Design review of the part built by this model. Coordinates are the model's own, in mm. Face numbers are marked on the shaded views. A direction names the side the tool comes from. Coordinates: 2 decimals unless noted, no trailing zeros. Order: outer loops, then holes, each group sorted by start corner. A loop starts at its lowest first (then second) coordinate and runs counter-clockwise, first axis right, second up. Notation, with made-up numbers: M 21,83 L 75,83 A10 cw 75,96 Z; hole C 61,-1 d8. An arc over 180 degrees is marked long. Use CSV: the item, a comma, the result in double quotes.
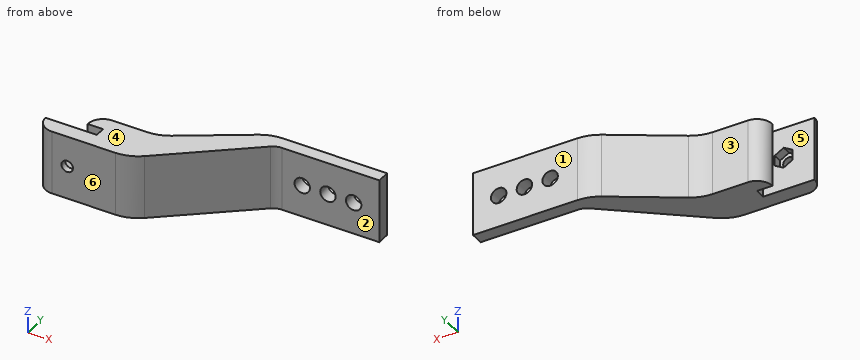
Autodesk Fusion 360 part; units mm, degrees
sketch "Sketch1" plane through (0, 0, 0) normal (0, 0, 1) x (1, 0, 0)
  line L0 (0, 0) -> (0, 6)
  line L1 (0, 6) -> (20, 6)
  line L2 (20, 6) -> (20, 10)
  line L3 (20, 10) -> (14, 10)
  line L4 (14, 16) -> (14, 10)
  line L5 (14, 16) -> (38, 16)
  line L6 (38, 16) -> (70, 36)
  line L7 (70, 36) -> (115, 36)
  line L8 (115, 36) -> (115, 31)
  line L9 (115, 31) -> (75, 31)
  line L10 (75, 31) -> (36, 0)
  line L11 (36, 0) -> (0, 0)
  dimension "d1" = 4
  dimension "d2" = 24
  dimension "d6" = 115
  dimension "d7" = 5
  dimension "d8" = 45
  dimension "d10" = 20
  dimension "d11" = 36
  dimension "d12" = 16
  dimension "d13" = 6
  dimension "d14" = 14
  dimension "d15" = 36
  dimension "d16" = 40
extrude "Extrude1" add sketch "Sketch1" along normal blind 25
sketch "Sketch2" plane through (0, 6, 0) normal (0, 1, 0) x (-1, 0, 0)
  line L0 (-20, 0) -> (0, 0)
  line L1 (0, 0) -> (0, 25)
  line L2 (0, 25) -> (-20, 25)
  line L3 (-20, 25) -> (-20, 0)
  line L4 (0, 13) -> (-20, 13) construction
  line L5 (-12, 25) -> (-12, 0) construction
  line L6 (-8.5, 15.0207) -> (-12, 17.0415)
  line L7 (-12, 17.0415) -> (-15.5, 15.0207)
  line L8 (-15.5, 15.0207) -> (-15.5, 10.9793)
  line L9 (-15.5, 10.9793) -> (-12, 8.9585)
  line L10 (-12, 8.9585) -> (-8.5, 10.9793)
  line L11 (-8.5, 10.9793) -> (-8.5, 15.0207)
  point P0 (-12, 13)
  dimension "d19" = 12
  dimension "d20" = 3.5
extrude "Extrude2" cut sketch "Sketch2" against normal blind 3.5 contours L6 L7 L8 L9 L10 L11
hole "Hole1" at (12, 6, 13) direction (0, -1, 0) diameter 4.5 end through all
sketch "Sketch3" plane through (0, 36, 0) normal (0, 1, 0) x (-1, 0, 0)
  line L0 (-115, 0) -> (-70, 0)
  line L1 (-70, 0) -> (-70, 25)
  line L2 (-70, 25) -> (-115, 25)
  line L3 (-115, 25) -> (-115, 0)
  line L4 (-115, 12.5) -> (-70, 12.5) construction
  line L5 (-105, 25) -> (-105, 0) construction
  point P0 (-105, 12.5)
  dimension "d26" = 10
hole "Hole2" at (105, 36, 12.5) direction (0, -1, 0) diameter 6 depth 6.5 tip angle 118
pattern_linear "R-Pattern1" count 3 spacing 10 along (-1, 0, 0) of "Hole2"
fillet "Fillet1" radius 15 1 edges at (70, 36, 12.5)
fillet "Fillet1" radius 6 1 edges at (75, 31, 12.5)
fillet "Fillet2" radius 15 2 edges at (38, 16, 12.5) (36, 0, 12.5)
fillet "Fillet3" radius 6 1 edges at (14, 16, 12.5)
fillet "Fillet4" radius 6 1 edges at (0, 0, 12.5)
(1) The part is to be moulded in two halves that separate along Y. For the marked faces 4, 5 and 6, say which applies: pulls with the +Y half, pulls with the -Y half, needs draft (parallel to the pull), parting line crosses it, or undercut.
The answers:
face 4,"needs draft"
face 5,"undercut"
face 6,"pulls with the -Y half"
(2) Wall thickness on probe 1 along Z at (x, y) = (95, 33); probe 2 along Z at (x, y) = (12, 1); probe 3 along X at (y, z) = (33.95, 12.5): over which ranges is each line inside the solid? List them lowest first.
The answers:
probe 1,"z = 0 to 9.5, 15.5 to 25"
probe 2,"z = 0 to 10.75, 15.25 to 25"
probe 3,"x = 66.73 to 82, 88 to 92, 98 to 102, 108 to 115"
(3) For the marked faces 1, 2 and 3, list the 3-axis set-ups (+Z, -Z, +X, -X, +Y, -Y) from which the entire face can be reached by the end or side of a thin tool; tool diameter is ignored.
The answers:
face 1,"+Z, -Z, +X, -X, +Y"
face 2,"+Z, -Z, +X, -Y"
face 3,"+Z, -Z, -X, +Y"
(4) Add section D-D on z = 12.5. Give the number of separate pieces and of enclosed holes in the cut face, and give its area (3 significant figures).
The answers:
separate pieces,"5"
enclosed holes,"0"
area,"908 mm2"
(5) Add section B-B on y = 32. State the section outline as (x, z) points, and give its area (3 significant figures).
The answers:
outline,"M 63.6,0 L 115,0 L 115,25 L 63.6,25 Z; hole C 85,12.5 d6; hole C 95,12.5 d6; hole C 105,12.5 d6"
area,"1,200 mm2"
(6) Clearance check with flat-ended pins moving along their axes: P1, Ø8, axis at x = 69.5, z = 6, coming from the +Y side; P2, Ø1, axis at x = 42, z = 3, coming from the +Y side; P3, Ø1.5, axis at y = 11.5, z = 6.5, coming from the +X side. State where each tip first meets the part, or that it passes through.
The answers:
P1,"stops at y = 35.98"
P2,"stops at y = 18.81"
P3,"stops at x = 51.41"
(7) Add section A-A on x = 85. State the section outline as (y, z) points, and give its area (3 significant figures).
The answers:
outline,"M 31,0 L 36,0 L 36,9.5 L 31,9.5 Z; M 31,15.5 L 36,15.5 L 36,25 L 31,25 Z"
area,"95.0 mm2"
